The model under review builds one solid part; all positions refer to its coordinate system, in mm. Give positions to 0.01 mm unless a question says otherwise; leave off trailing zeros. Order: outer loops, then holes, each group sorted by start corner. A loop starts at its lowest first (then second) coordinate and runs counter-clockwise, first axis right, second up. Notation, with made-up numbers: (72.25, 58.25) - (77.25, 58.25) arc R28 cw to (77.25, 76.25) - close; hole circle Ø9 at (17.5, -39.75). An arc over 180 degrees is marked (long way). Write item = value, one per line. Start each with the question number.
1. We need section A-A, the plane y = 190.5. Give the boundary of the cut face in (x, z).
2. Wall thickness on probe 1 along Z at (x, y) = (-327, 190.5); probe 2 along X at (y, z) = (191.75, 80): over which ranges is each line inside the solid? List them lowest first.
3. We need section B-B, the plane z = 23.5. Give the boundary of the cut face in (x, y), and give its area (3 significant figures).
4. For P1, Ø1.9, axis at x = -353.5, y = 190, coming from the -Z side; P2, Ø3, axis at y = 191.5, z = 89.5, coming from the -X side; P3, Ø3, axis at y = 192.5, z = 11.5, coming from the +X side, all flat-tipped, find the tip position at first contact; note any pin that passes through.
5. We need section C-C, the plane x = 199. Give the boundary of the cut face in (y, z).
Autodesk Inventor part; units mm, degrees
ref_plane "YZ Plane" through (0, 0, 0) normal (1, 0, 0) x (0, 1, 0)
ref_plane "XZ Plane" through (0, 0, 0) normal (0, 1, 0) x (-1, 0, 0)
ref_plane "XY Plane" through (0, 0, 0) normal (0, 0, 1) x (1, 0, 0)
sketch "Sketch1" plane through (0, 0, 0) normal (0, 0, 1) x (1, 0, 0)
  line L0 (-379.6568, 188.1861) -> (255.3432, 188.1861)
  line L1 (255.3432, 188.1861) -> (255.3432, 194.5361)
  line L2 (255.3432, 194.5361) -> (-379.6568, 194.5361)
  line L3 (-379.6568, 194.5361) -> (-379.6568, 188.1861)
  point P0 (0, 0)
  dimension "d0" = 635
  dimension "d1" = 6.35
extrude "Extrusion1" add sketch "Sketch1" along normal blind 355.6
sketch "Sketch2" plane through (-379.6568, 188.1861, 0) normal (0, -1, 0) x (1, 0, 0)
  line L0 (635, 355.6) -> (0, 355.6)
  line L1 (0, 0) -> (0, 355.6)
  line L2 (0, 0) -> (635, 0)
  line L3 (635, 0) -> (635, 355.6)
  line L4 (12.7, 355.6) -> (622.3, 355.6)
  line L5 (622.3, 355.6) -> (622.3, 0)
  line L6 (622.3, 0) -> (12.7, 0)
  line L7 (12.7, 0) -> (12.7, 355.6)
  point P0 (379.6568, 0)
  dimension "d4" = 609.6
  dimension "d5" = 355.6
  dimension "d6" = 12.7
extrude "Extrusion2" cut sketch "Sketch2" against normal blind 355.6 contours L3 L2 L5 L0 | L7 L2 L1 L0
sketch "Sketch3" plane through (-366.9568, 194.5361, 0) normal (0, 1, 0) x (1, 0, 0)
  line L0 (0, 0) -> (0, -355.6)
  line L1 (609.6, 0) -> (558.8, 0)
  line L2 (558.8, 0) -> (558.8, -31.75)
  line L3 (558.8, -31.75) -> (609.6, -31.75)
  line L4 (609.6, -31.75) -> (609.6, 0)
  line L5 (0, 0) -> (50.8, 0)
  line L6 (50.8, 0) -> (50.8, -31.75)
  line L7 (50.8, -31.75) -> (0, -31.75)
  line L8 (0, -31.75) -> (0, 0)
  line L9 (0, -133.35) -> (38.1, -133.35)
  line L10 (38.1, -133.35) -> (38.1, -31.75)
  line L11 (38.1, -31.75) -> (0, -31.75)
  line L12 (0, -31.75) -> (0, -133.35)
  point P0 (366.9568, 0)
  dimension "d9" = 50.8
  dimension "d10" = 31.75
  dimension "d11" = 50.8
  dimension "d12" = 31.75
  dimension "d13" = 38.1
  dimension "d14" = 101.6
extrude "Extrusion3" cut sketch "Sketch3" against normal blind 25.4
properties part number "24in-by-14in_electronics_board"
Model answer:
q1.outline = (-366.96, 133.35) - (-328.86, 133.35) - (-328.86, 31.75) - (-316.16, 31.75) - (-316.16, 0) - (191.84, 0) - (191.84, 31.75) - (242.64, 31.75) - (242.64, 355.6) - (-366.96, 355.6) - close
q2.probe_1 = 31.75 to 355.6
q2.probe_2 = -328.86 to 242.64
q3.outline = (-316.16, 188.19) - (191.84, 188.19) - (191.84, 194.54) - (-316.16, 194.54) - close
q3.area = 3,230 mm2
q4.P1 = 133.35
q4.P2 = -328.86
q4.P3 = 191.84
q5.outline = (188.19, 31.75) - (194.54, 31.75) - (194.54, 355.6) - (188.19, 355.6) - close
